Design review of the part built by this model. Coordinates are the model's own, in mm. A direction names the side the tool comes from. Coordinates: 2 decimals unless noted, no trailing zeros. Loops run counter-clockwise (first coordinate to the right, second up) from the corner with the lowest first, then second, coordinate; pieces in that order, holes last. Notation, with made-up numbers: M -40,-3 L 15,-3 A10 ccw 15,14 Z; hole C -20.75,89.25 d11. An arc over 180 degrees is marked long. Answer as a JSON object with one key per item and string values. Group by question number.
1. Insertion check: pin 1 (6 mm diameter, centred on y = 11.5, z = 12.5, fed in from -X); pin 2 (3 mm diameter, centred on x = 6, z = 10, fed in from +Y); pin 3 (5 mm diameter, centred on x = 7.5, y = 13.6, fed in from +Z). Each pin has a flat end and moves straight along its axis. Give the tip position at first contact, or say it passes through.
2. Machinability: for faces 5 (the flat face through (0, -8, 1.45)), 6 (the flat face through (0, 14, 1.45)), 7 (the cylindrical face through (-7.836, -2.109, 4.088)), which of the approach directions +Z, -Z, +X, -X, +Y, -Y give a long, thin tool a straight path to every point of the face, cutting with its end or side? Answer none if there is none.
3. Consider section D-D (y = -10). State the section outline as (x, z) points (3 decimals).
4. Consider section B-B (x = 0). State the section outline as (y, z) points (3 decimals).
5. Consider section A-A (y = -13.6). State the section outline as (x, z) points (3 decimals), then the cut area to 3 significant figures.
6. To check wall thickness, follow probe 1 along Y at (x, z) = (-7.5, 0.7) (3 decimals); probe 2 along Z at (x, y) = (-5, -4.5); probe 3 along Z at (x, y) = (6.75, -11.5). State the ranges of each line that lie inside material, in increasing order.
7. Consider section C-C (x = 8.75). State the section outline as (y, z) points (3 decimals), then the cut area to 3 significant figures.
8. Draft analysis for pull direction Y (two halves, no side actions). For faces 1 (the flat face through (-3.7, -3.4, 6.8)), 2 (the cylindrical face through (-7.71, 15.21, 0.74)), 3 (the cylindrical face through (-1.041, 11.832, 10.498)), 4 (the cylindrical face through (7.29, 15.21, 0.74)), state which applies: +Y half, -Y half, draft (parallel to the pull), parting line (faces both ways), or undercut.
from build123d import *

# Parameters (mm, degrees)
SKETCH1_W           = 19.75
SKETCH1_H           = 31.95
BOSS_EXTRUDE1_DEPTH = 1.45
SKETCH2_R           = 1.625
CUT_EXTRUDE1_DEPTH  = 2.45
SKETCH3_R           = 9.875
BOSS_EXTRUDE2_DEPTH = 5.35
SKETCH4_R           = 8
BOSS_EXTRUDE3_DEPTH = 9.5
FILLET1_R           = 2


with BuildPart() as part:
    # Sketch1 → Boss-Extrude1 (new body)
    with BuildSketch(Plane.XY):
        Rectangle(SKETCH1_W, SKETCH1_H)
    extrude(amount=BOSS_EXTRUDE1_DEPTH)

    # Sketch2 → Cut-Extrude1 (cut, through all)
    with BuildSketch(Plane.XY.offset(1.45)):
        with Locations((-7.5, 13.6)):
            Circle(SKETCH2_R)
        with Locations((-7.5, -13.6)):
            Circle(SKETCH2_R)
        with Locations((7.5, -13.6)):
            Circle(SKETCH2_R)
        with Locations((7.5, 13.6)):
            Circle(SKETCH2_R)
    extrude(amount=-CUT_EXTRUDE1_DEPTH, mode=Mode.SUBTRACT)

    # Sketch3 → Boss-Extrude2 (add)
    with BuildSketch(Plane.XY.offset(1.45)):
        with Locations((0, 3.9)):
            Circle(SKETCH3_R)
    extrude(amount=BOSS_EXTRUDE2_DEPTH)

    # Sketch4 → Boss-Extrude3 (add)
    with BuildSketch(Plane.XY.offset(6.8)):
        with Locations((0, 3.9)):
            Circle(SKETCH4_R)
    extrude(amount=BOSS_EXTRUDE3_DEPTH)

    # Fillet1
    fillet1_edges = [part.edges().sort_by_distance(p)[0] for p in [
        (-8, 3.9, 16.3),
    ]]
    fillet(fillet1_edges, radius=FILLET1_R)


solid = part.part
Findings below:
{
 "1": {"pin 1": "stops at x = -6.55", "pin 2": "stops at y = 10.51", "pin 3": "stops at z = 6.8"},
 "2": {"face 5": "+Z, -Y", "face 6": "+Z, +Y", "face 7": "+Z"},
 "3": {"outline": "M -9.875,0 L 9.875,0 L 9.875,1.45 L -9.875,1.45 Z"},
 "4": {"outline": "M -15.975,0 L 15.975,0 L 15.975,1.45 L 13.775,1.45 L 13.775,6.8 L 11.9,6.8 L 11.9,14.3 A2 ccw 9.9,16.3 L -2.1,16.3 A2 ccw -4.1,14.3 L -4.1,6.8 L -5.975,6.8 L -5.975,1.45 L -15.975,1.45 Z"},
 "5": {"outline": "M -9.875,0 L -9.125,0 L -9.125,1.45 L -9.875,1.45 Z; M -5.875,0 L 5.875,0 L 5.875,1.45 L -5.875,1.45 Z; M 9.125,0 L 9.875,0 L 9.875,1.45 L 9.125,1.45 Z", "area": "19.2 mm^2"},
 "6": {"probe 1": "y = -15.975 to -15.225, -11.975 to 11.975, 15.225 to 15.975", "probe 2": "z = 0 to 6.8", "probe 3": "z = 0 to 1.45"},
 "7": {"outline": "M -15.975,0 L -14.638,0 L -14.638,1.45 L -15.975,1.45 Z; M -12.562,0 L 12.562,0 L 12.562,1.45 L 8.477,1.45 L 8.477,6.8 L -0.677,6.8 L -0.677,1.45 L -12.562,1.45 Z; M 14.638,0 L 15.975,0 L 15.975,1.45 L 14.638,1.45 Z", "area": "89.3 mm^2"},
 "8": {"face 1": "draft", "face 2": "undercut", "face 3": "parting line", "face 4": "undercut"}
}
